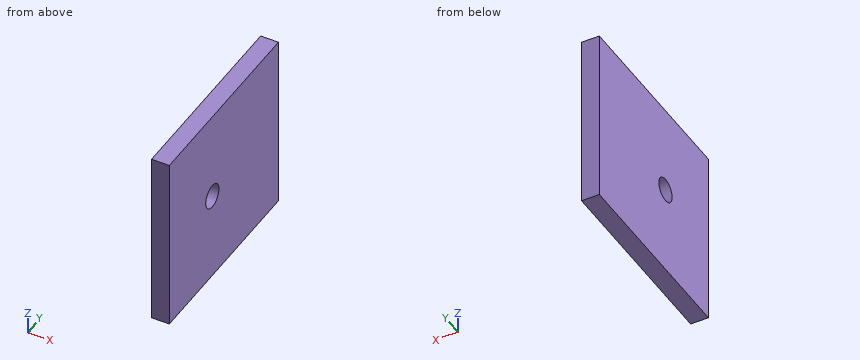
from build123d import *

# Parameters (mm, degrees)
SKETCH_1_W          = 30
SKETCH_1_H          = 40
EXTRUDE_1_DEPTH     = 3
SKETCH_2_R          = 2
CUT_EXTRUDE_1_DEPTH = 4
SKETCH_3_W          = 30
SKETCH_3_H          = 7
CUT_EXTRUDE_2_DEPTH = 4


with BuildPart() as part:
    # 草图1 → 凸台-拉伸1 (new body)
    with BuildSketch(Plane(origin=(0, 0, 0), x_dir=(0, 0, -1), z_dir=(1, 0, 0))):
        Rectangle(SKETCH_1_W, SKETCH_1_H)
    extrude(amount=EXTRUDE_1_DEPTH)

    # 草图2 → 切除-拉伸1 (cut, through all)
    with BuildSketch(Plane(origin=(3, 0, 0), x_dir=(0, 0, -1), z_dir=(1, 0, 0))):
        Circle(SKETCH_2_R)
    extrude(amount=-CUT_EXTRUDE_1_DEPTH, mode=Mode.SUBTRACT)

    # 草图3 → 切除-拉伸2 (cut, through all)
    with BuildSketch(Plane.ZY):
        with Locations((0, -16.5)):
            Rectangle(SKETCH_3_W, SKETCH_3_H)
    extrude(amount=-CUT_EXTRUDE_2_DEPTH, mode=Mode.SUBTRACT)


solid = part.part
Source: CAD feature listing. Evaluate the final solid. Frame: model axes, mm. Round coordinates to 2 decimals unless told otherwise and drop trailing zeros. Write each loop counter-clockwise with the first axis right and the second up, starting at its lowest first coordinate (ties: lowest second). Pieces come first, ordered by that corner, then holes. Notation, with made-up numbers: M 58.5,8.5 L 107.5,8.5 A12 cw 107.5,21.5 Z; hole C 76.25,5 d11. An arc over 180 degrees is marked long. One line per item, written item: value. Start each with the question number.
Item 1: Section query A-A (z = 0). Return the cut outline in (x, y), plus the area to 3 significant figures.
Item 2: Ray query, L1, parallel to Y at x = 1.4, z = 0; L2, parallel to Z at x = 1.9, y = 1; L3, parallel to Z at x = 1.95, y = 1.5. Return the intervals inside material, ascending. Write a range as from..to.
Item 3: Section query B-B (y = 0). Return the cut outline in (x, z).
Result set:
1. outline: M 0,-13 L 3,-13 L 3,-2 L 0,-2 Z; M 0,2 L 3,2 L 3,20 L 0,20 Z
1. area: 87.0 mm²
2. L1: y = -13..-2, 2..20
2. L2: z = -15..-1.73, 1.73..15
2. L3: z = -15..-1.32, 1.32..15
3. outline: M 0,-15 L 3,-15 L 3,-2 L 0,-2 Z; M 0,2 L 3,2 L 3,15 L 0,15 Z
